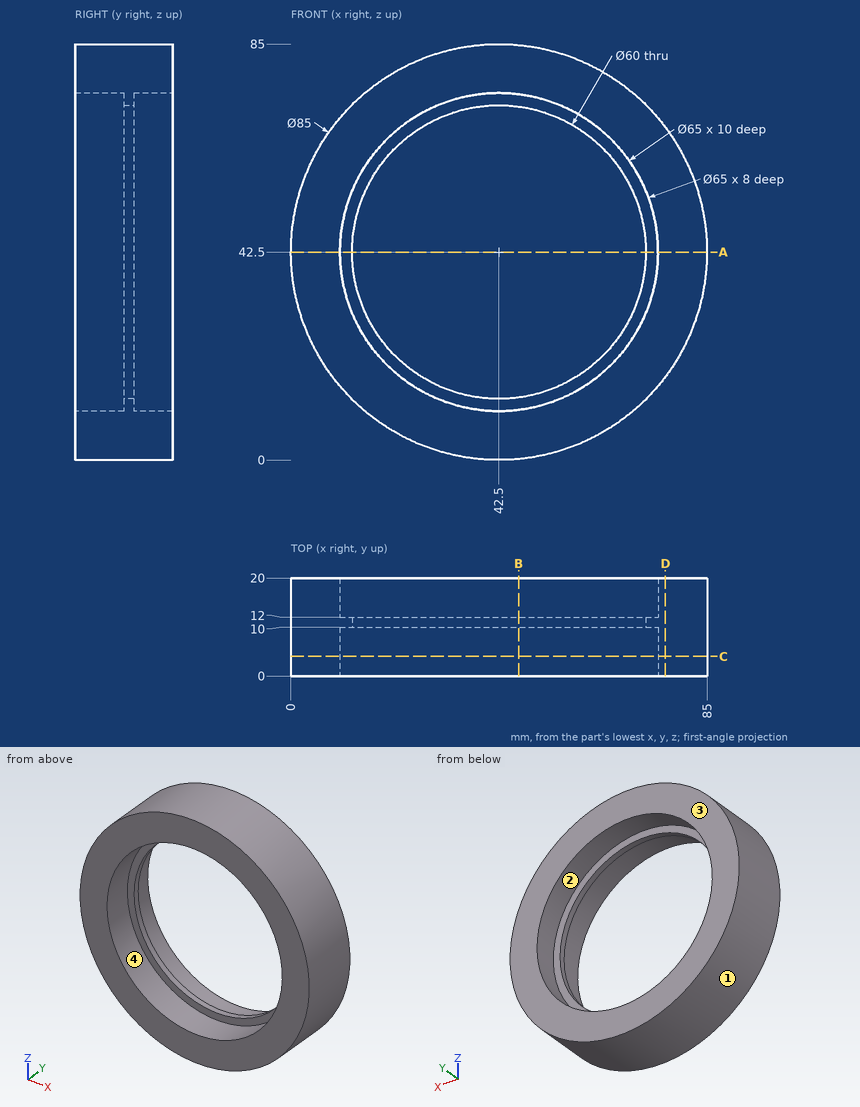
For this review, use the dimensioned drawing (mm, ordinates from the lowest corner) and the shaded views. Give positions to 0.01 mm unless a question says otherwise; leave off trailing zeros. Write each loop counter-clockwise with the first axis right and the second up, starting at its lowest first coordinate (ties: lowest second). Pieces come first, ordered by that corner, then holes.
(1) Consider section C-C, the plane y = 4. Give the boundary of the cut face in (x, z), and give its area (3 significant figures).
(2) Consider section D-D, the plane x = 76.5. Give the boundary of the cut face in (y, z).
(3) Consider section B-B, the plane x = 46.5. Give the boundary of the cut face in (y, z), and give its area (3 significant figures).
(4) The part is to be moulded in two halves that separate along Z. For the marked faces 1, 2, 3 and 4, say which applies: released by +Z, released by -Z, zero draft, split by the parting line, or undercut.
(5) Consider section A-A, the plane z = 42.5. Give the boundary of the cut face in (x, y), and give its area (3 significant figures).
(6) To check wall thickness, follow L1, parallel to X at y = 17.5, z = 42.5; L2, parallel to X at y = 11.5, z = 42.5. State the ranges of each line that lie inside material, in increasing order.
(7) For P1, Ø5, axis at x = 29.5, y = 10, coming from the -Z side; P2, Ø8, axis at y = 8.5, z = 12, coming from the -X side; P3, Ø2, axis at y = 6, z = 38.5, coming from the -X side; P4, Ø12, axis at x = 13.5, z = 74.5, coming from the +Y side, all flat-tipped, find the tip position at first contact; note any pin that passes through.
Returned:
1. outline: circle Ø85 at (42.5, 42.5); hole circle Ø65 at (42.5, 42.5)
1. area: 2,360 mm2
2. outline: (0, 17) - (20, 17) - (20, 68) - (0, 68) - close
3. outline: (0, 0.19) - (20, 0.19) - (20, 10.25) - (12, 10.25) - (12, 12.77) - (10, 12.77) - (10, 10.25) - (0, 10.25) - close; (0, 74.75) - (10, 74.75) - (10, 72.23) - (12, 72.23) - (12, 74.75) - (20, 74.75) - (20, 84.81) - (0, 84.81) - close
3. area: 412 mm2
4. face 1: split by the parting line
4. face 2: undercut
4. face 3: zero draft
4. face 4: undercut
5. outline: (0, 0) - (10, 0) - (10, 10) - (12.5, 10) - (12.5, 12) - (10, 12) - (10, 20) - (0, 20) - close; (72.5, 10) - (75, 10) - (75, 0) - (85, 0) - (85, 20) - (75, 20) - (75, 12) - (72.5, 12) - close
5. area: 410 mm2
6. L1: x = 0 to 10, 75 to 85
6. L2: x = 0 to 12.5, 72.5 to 85
7. P1: stops at z = 1.32
7. P2: stops at x = 9.27
7. P3: stops at x = 0.11
7. P4: stops at y = 20
